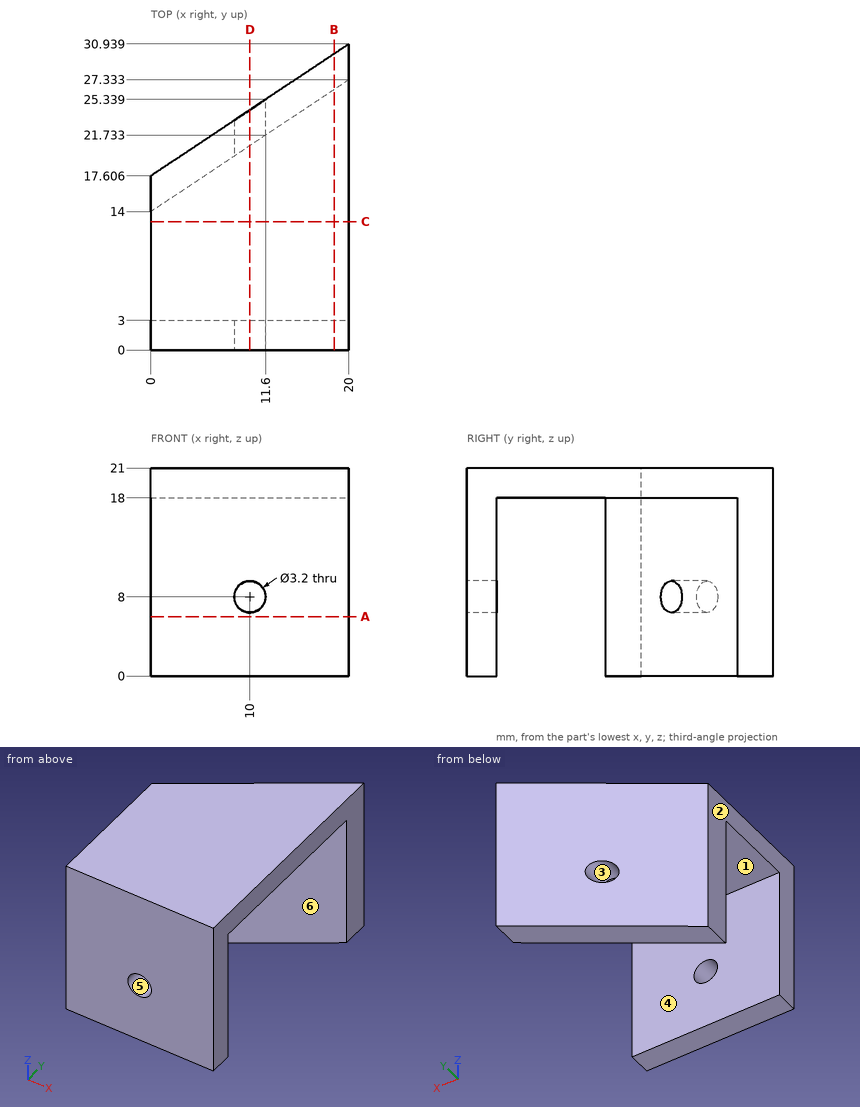
Answer from the drawing. Dimensions are ordinates in mm from the lowest x, y and z of the part. A direction names the side the tool comes from. Round coordinates to 2 decimals unless told otherwise and drop trailing zeros. Loops run counter-clockwise (first coordinate to the right, second up) from the corner with the lowest first, then second, coordinate; pieces in that order, holes last. Notation, with made-up numbers: M 77.5,20.25 L 82.5,20.25 A32 cw 82.5,57.25 Z; hole C 46,47 d8. An arc over 180 degrees is marked long. One line per question, with ' | ' between items. Start each with the question number.
(1) A cutting plane is placed at C-C on y = 13. Write down the section's boundary in (x, z).
(2) A cutting plane is placed at A-A on z = 6. Write down the section's boundary in (x, y) (1 decimal), plus the area to 3 significant figures.
(3) Flat-ended cylindrical pins translate along their axes: pin 1 Ø6 at (x, y) = (14.5, 15.5) entering from -Z; pin 2 Ø6 at (x, y) = (13, 4) entering from -Z; pin 3 Ø5 at (x, z) = (10, 8) entering from +Y; pin 4 Ø9 at (x, z) = (13.5, 7.5) entering from +Y (1 decimal). Find the tip coordinate at first contact, or state that the pin passes through.
(4) A cutting plane is placed at B-B on x = 18.5. Write down the section's boundary in (y, z), plus the area to 3 significant figures.
(5) Find the intervals of material crossed by line 1 (Z direction, x = 10, y = 2.3); line 2 (Y direction, x = 1, z = 7) (1 decimal); line 3 (Z direction, x = 2, y = 11.5), in increasing order.
(6) For a pull along X with two mould halves and no side action, classify the marked faces 1, 2 and 3 as released by +X, released by -X, zero draft, split by the parting line, or undercut.
(7) A tool of negligible diameter and unlimited length cuts with its end or side. For the marked faces 4, 5 and 6, from which of +Z, -Z, +X, -X, +Y, -Y can it reach the whole face along a straight path? Write none if from no direction.
(8) A cutting plane is placed at D-D on x = 10. Write down the section's boundary in (y, z).
Geometry check:
1) outline: M 0,18 L 20,18 L 20,21 L 0,21 Z
2) outline: M 0,0 L 20,0 L 20,3 L 0,3 Z; M 0,14 L 20,27.3 L 20,30.9 L 0,17.6 Z | area: 132 mm²
3) pin 1: stops at z = 18 | pin 2: stops at z = 0 | pin 3: stops at y = 25.94 | pin 4: stops at y = 29.6
4) outline: M 0,0 L 3,0 L 3,18 L 26.33,18 L 26.33,0 L 29.94,0 L 29.94,21 L 0,21 Z | area: 209 mm²
5) line 1: z = 0 to 6.4, 9.6 to 21 | line 2: y = 0 to 3, 14.7 to 18.3 | line 3: z = 18 to 21
6) face 1: zero draft | face 2: released by -X | face 3: undercut
7) face 4: -Z, +X, -X | face 5: +Y, -Y | face 6: -Z, +X
8) outline: M 0,0 L 3,0 L 3,6.4 L 0,6.4 Z; M 0,9.6 L 3,9.6 L 3,18 L 20.67,18 L 20.67,9.6 L 24.27,9.6 L 24.27,21 L 0,21 Z; M 20.67,0 L 24.27,0 L 24.27,6.4 L 20.67,6.4 Z
